The figure shows three views and two pictorial views of one solid part (mm, origin at its lowest corner). Answer the questions. A direction names the side the tool comes from. Coordinates: 2 decimals unless noted, no trailing zeros. Order: outer loops, then holes, each group sorted by start corner. A loop starts at its lowest first (then second) coordinate and runs counter-clockwise, first axis right, second up. Notation, with made-up numbers: (11, 72.5) -> (36, 72.5) arc R21 ccw to (36, 80.5) -> close; hole circle Ø5 at (52, 23.25). An arc over 180 degrees is marked (long way). Write item = value, one per line.
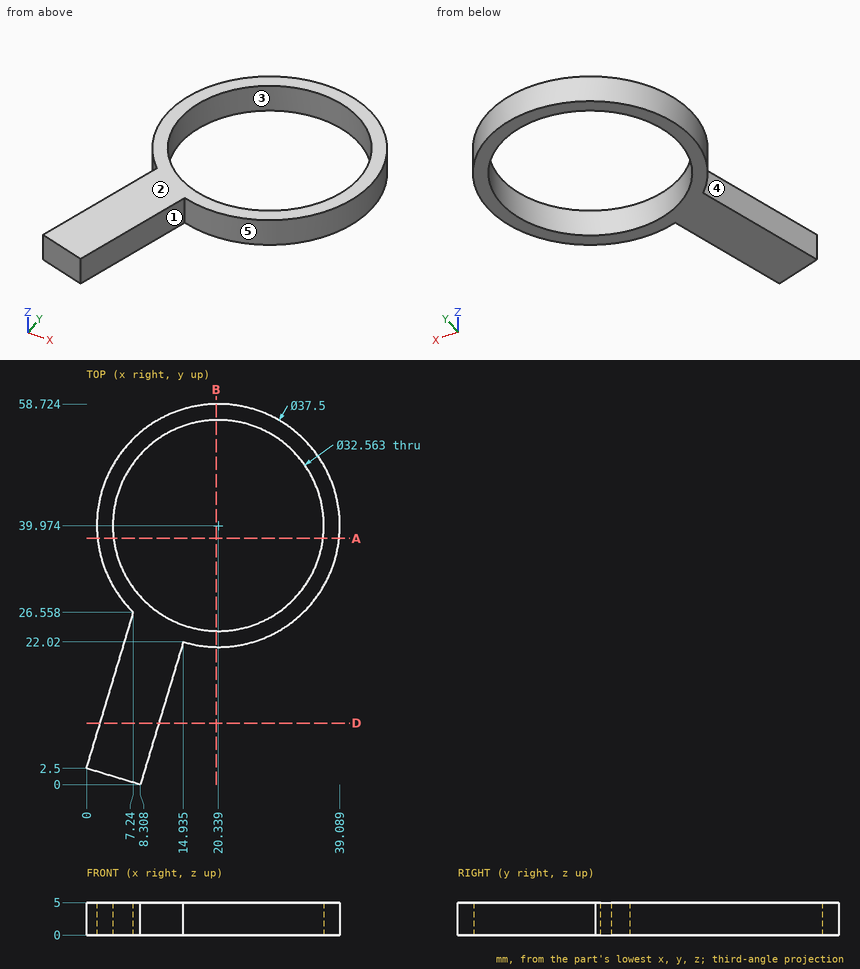
Q1. Each of these flat-tipped pins is pushed along its axis until it touches: pin 1 Ø3 at (y, z) = (47, 2) entering from +X (1 decimal); pin 2 Ø3 at (x, y) = (26, 26) entering from -Z; pin 3 Ø3 at (x, z) = (11.5, 3) entering from +Y. Where does it stop, or does it pass through?
The answers:
pin_1 = 38.3
pin_2 = 0
pin_3 = 57.23
Q2. Section B-B, the plane x = 20 is taken. Give the vertices of the cut face in (y, z), plus the area to 3 significant figures.
The answers:
outline = (21.23, 0) -> (23.7, 0) -> (23.7, 5) -> (21.23, 5) -> close; (56.25, 0) -> (58.72, 0) -> (58.72, 5) -> (56.25, 5) -> close
area = 24.7 mm2
Q3. Section A-A, the plane y = 38 is taken. Give the vertices of the cut face in (x, z) (1 decimal).
The answers:
outline = (1.7, 0) -> (4.2, 0) -> (4.2, 5) -> (1.7, 5) -> close; (36.5, 0) -> (39, 0) -> (39, 5) -> (36.5, 5) -> close
Q4. Section D-D, the plane y = 9.5 is taken. Give the vertices of the cut face in (x, z).
The answers:
outline = (2.11, 0) -> (11.17, 0) -> (11.17, 5) -> (2.11, 5) -> close
Q5. The mould has two halves that part along Y. Classify the marked faces 1, 2 and 3: released by +Y, released by -Y, zero draft, split by the parting line, or undercut.
The answers:
face_1 = released by -Y
face_2 = zero draft
face_3 = undercut
Q6. A tool of negligible diameter and unlimited length cuts with its end or side. For the marked faces 4 and 5, from which of +Z, -Z, +X, -X, +Y, -Y can it reach the whole face along a straight path? Write none if from no direction.
The answers:
face_4 = +Z, -Z, -X
face_5 = +Z, -Z
Q7. Find the intervals of material crossed by line 1 along X through (y, z) = (42.5, 2.25) (1 decimal); line 2 along Y through (x, z) = (24.5, 3.2) (1 decimal); line 3 along X through (y, z) = (31, 1.65) (1 decimal), in increasing order.
The answers:
line_1 = 1.8 to 4.3, 36.4 to 38.9
line_2 = 21.7 to 24.2, 55.7 to 58.3
line_3 = 3.9 to 6.8, 33.9 to 36.8
